Source: CAD feature listing. Evaluate the final solid. Frame: model axes, mm. Face numbers are marked on the shaded views. A direction names the side the tool comes from. Coordinates: 2 decimals unless noted, no trailing zeros. Order: outer loops, then holes, each group sorted by start corner. A loop starts at its lowest first (then second) coordinate and runs counter-clockwise, first axis right, second up.
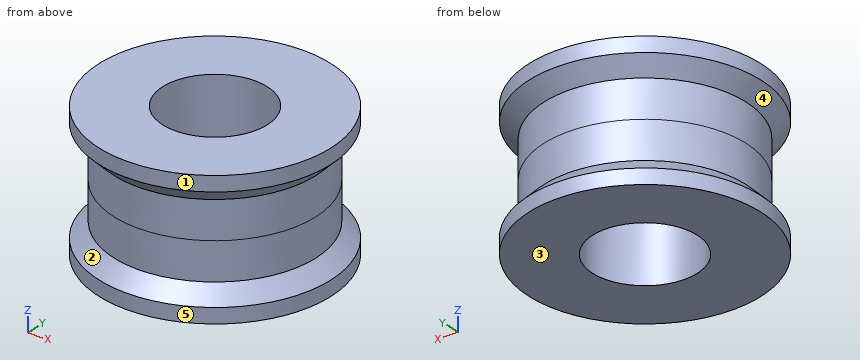
```python
from build123d import *

# Parameters (mm, degrees)
SKETCH1_R           = 7.75
SKETCH1_R_2         = 3.5
BOSS_EXTRUDE1_DEPTH = 1
SKETCH2_R           = 6.75
SKETCH2_R_2         = 3.5
BOSS_EXTRUDE2_DEPTH = 3.5
CHAMFER1_SIZE       = 1


with BuildPart() as part:
    # Sketch1 → Boss-Extrude1 (new body)
    with BuildSketch(Plane.XY):
        Circle(SKETCH1_R)
        Circle(SKETCH1_R_2, mode=Mode.SUBTRACT)
    extrude(amount=BOSS_EXTRUDE1_DEPTH)

    # Sketch2 → Boss-Extrude2 (add)
    with BuildSketch(Plane.XY.offset(1)):
        Circle(SKETCH2_R)
        Circle(SKETCH2_R_2, mode=Mode.SUBTRACT)
    extrude(amount=BOSS_EXTRUDE2_DEPTH)

    # Chamfer1
    chamfer1_edges = [part.edges().sort_by_distance(p)[0] for p in [
        (-6.75, 0, 1),
    ]]
    chamfer(chamfer1_edges, length=CHAMFER1_SIZE - 0.0001)  # a hair under: the kernel refuses the full size

    # Mirror5: part across plane


with BuildPart() as part_1:
    add(part.part)
    add(part.part.mirror(Plane.XY.offset(4.5)))


solid = part_1.part
```
1. Section query C-C on z = 8.25. Return loops of the section in (x, y).
Findings:
outline: circle Ø15.5 at (0, 0); hole circle Ø7 at (0, 0)
2. Draft query along Z for the marked faces 3, 4 and 5. Return one class per face: released by +Z, released by -Z, zero draft, split by the parting line, or undercut.
Findings:
face 3: released by -Z
face 4: undercut
face 5: zero draft
3. Ray query, line 1 (Y direction, x = 0, z = 6.55); line 2 (Z direction, x = 6, y = -4.5); line 3 (Z direction, x = -6.25, y = 3.75). Return the intervals inside material, ascending.
Findings:
line 1: y = -6.75 to -3.5, 3.5 to 6.75
line 2: z = 0 to 1.25, 7.75 to 9
line 3: z = 0 to 1.46, 7.54 to 9
4. Pin query (flat end, axial travel): P1, Ø1.5, axis at y = 0, z = 7, coming from the +X side; P2, Ø2, axis at y = -5.5, z = 5, coming from the +X side; P3, Ø3, axis at y = 2.5, z = 4.5, coming from the +X side. Return the tip coordinate at first contact, or that it passes through.
Findings:
P1: stops at x = 7.5
P2: stops at x = 5.03
P3: stops at x = 6.68
5. Access query for the marked faces 1 and 2. Directions: +Z, -Z, +X, -X, +Y, -Y. A direction counts if a zero-diameter tool reaches every point of the face in a straight line with its end or side. Return the directions, or none.
Findings:
face 1: +Z, -Z
face 2: none
6. Section query D-D on z = 4.75. Return loops of the section in (x, y), plus the area to 3 significant figures.
Findings:
outline: circle Ø13.5 at (0, 0); hole circle Ø7 at (0, 0)
area: 105 mm2
